```python
from build123d import *

# Parameters (mm, degrees)
F1_DEPTH = 38.1
F2_R     = 9.561336
F3_DEPTH = 50.8
F4_R     = 3.317837
F5_DEPTH = 42.926
F6_W     = 103.955641
F6_H     = 24.375808
F7_DEPTH = 50.8
F8_R     = 2.876859
F9_DEPTH = 45.212


with BuildPart() as f1:
    # F0 (on Front) → F1 (new body)
    with BuildSketch(Plane.XZ):
        Polygon((0, 74.93), (0, 0), (304.8, 0), (304.8, 19.05), align=None)
    extrude(amount=F1_DEPTH)

    # F2 (on face) → F3 (cut)
    with BuildSketch(Plane(origin=(0, 0, 0), x_dir=(0, -1, 0), z_dir=(-1, 0, 0))):
        with Locations((18.415, 39.243001)):
            Circle(F2_R)
    extrude(amount=-F3_DEPTH, mode=Mode.SUBTRACT)

    # F4 (on face) → F5 (cut)
    with BuildSketch(Plane(origin=(0, 0, 0), x_dir=(-1, 0, 0), z_dir=(0, 1, 0))):
        with Locations((-24.803754, 13.480514)):
            Circle(F4_R)
    extrude(amount=-F5_DEPTH, mode=Mode.SUBTRACT)

    # F6 (on face) → F7 (cut)
    with BuildSketch(Plane.XZ.offset(38.1)):
        with Locations((138.49657, 18.819557)):
            Rectangle(F6_W, F6_H)
    extrude(amount=-F7_DEPTH, mode=Mode.SUBTRACT)

    # F8 (on face) → F9 (cut)
    with BuildSketch(Plane.XZ.offset(38.1)):
        with Locations((295.173943, 5.17409)):
            Circle(F8_R)
    extrude(amount=-F9_DEPTH, mode=Mode.SUBTRACT)


solid = f1.part
```
The listing builds one solid part. Answer for the finished solid, in the listing's coordinates (mm). A direction names the side the tool comes from. Give positions to 0.01 mm unless a question says otherwise; leave off trailing zeros. Order: outer loops, then holes, each group sorted by start corner. A loop starts at its lowest first (then second) coordinate and runs counter-clockwise, first axis right, second up.
1) Determine the mould class of faces 4 (the face through (304.8, -19, 9)), 5 (the face through (292.3, -19.3, 5.3)), 6 (the face through (0, -23, 30)) for opening direction X: pulls with the +X half, pulls with the -X half, needs draft (parallel to the pull), parting line crosses it, or undercut.
Reported:
face 4: pulls with the +X half
face 5: undercut
face 6: pulls with the -X half
2) For faces 1 (the face through (150, -19, 0)), 2 (the face through (50.8, -18, 39)), 3 (the face through (138, -19, 6.632)), determine the directions among +Z, -Z, +X, -X, +Y, -Y from which every point of the face is accessible in a straight line to the end or side of a thin tool.
Reported:
face 1: -Z, +X, -X, +Y, -Y
face 2: -X
face 3: +Y, -Y
3) Consider line 1 along X through (y, z) = (-15.5, 18); line 2 along X through (y, z) = (-21, 14.5); line 3 along Y through (x, z) = (49.5, 47) (3 decimals). Determine where each line is inside the solid, lowest interval first.
Reported:
line 1: x = 0 to 86.52, 190.47 to 304.8
line 2: x = 0 to 21.65, 27.96 to 86.52, 190.47 to 304.8
line 3: y = -38.1 to -24.005, -12.825 to 0
4) Find section C-C on z = 43. Write down the section's boundary in (x, y).
Reported:
outline: (0, -38.1) - (174.16, -38.1) - (174.16, 0) - (0, 0) - (0, -9.62) - (50.8, -9.62) - (50.8, -27.21) - (0, -27.21) - close
5) Given P1, Ø8, axis at x = 125, y = -7.5, coming from the +Z side; P2, Ø6, axis at x = 192.5, y = -30.5, coming from the +Z side; P3, Ø5.5, axis at x = 24.8, z = 13.48, coming from the -Y side; P4, Ø5.5, axis at y = -14.5, z = 35, coming from the -X side, each flat-ended and moving along its own axis, determine where each tip first touches the part or whether it passes through.
Reported:
P1: stops at z = 52.75
P2: stops at z = 40.19
P3: passes through
P4: stops at x = 50.8
6) Find section A-A on x = 166.5. Write down the section's boundary in (y, z) (3 decimals), then the cut area to 3 significant figures.
Reported:
outline: (-38.1, 0) - (0, 0) - (0, 6.632) - (-38.1, 6.632) - close; (-38.1, 31.007) - (0, 31.007) - (0, 44.405) - (-38.1, 44.405) - close
area: 763 mm2
7) Find section B-B on y = -24. Write down the section's boundary in (x, z).
Reported:
outline: (0, 0) - (304.8, 0) - (304.8, 19.05) - (0, 74.93) - (0, 47) - (50.8, 47) - (50.8, 31.48) - (0, 31.48) - close; hole circle Ø6.64 at (24.8, 13.48); hole (86.52, 6.63) - (190.47, 6.63) - (190.47, 31.01) - (86.52, 31.01) - close; hole circle Ø5.75 at (295.17, 5.17)
8) Find section D-D on x = 107.5. Write down the section's boundary in (y, z).
Reported:
outline: (-38.1, 0) - (0, 0) - (0, 6.63) - (-38.1, 6.63) - close; (-38.1, 31.01) - (0, 31.01) - (0, 55.22) - (-38.1, 55.22) - close
